```python
from build123d import *

# Parameters (mm, degrees)
SKETCH1_W             = 88.9
SKETCH1_H             = 38.1
BOSS_EXTRUDE1_DEPTH   = 12.7
SKETCH2_W             = 19.05
SKETCH2_H             = 25.4
CUT_EXTRUDE2_DEPTH    = 50.99995
SKETCH5_W             = 31.496
SKETCH5_H             = 31.75
CUT_EXTRUDE3_DEPTH    = 50.99995
BOSS_EXTRUDE2_START   = -6.35
BOSS_EXTRUDE2_DEPTH   = 6.35
SKETCH7_W             = 6.604
SKETCH7_H             = 6.604
CUT_EXTRUDE4_DEPTH    = 1.27
F_4_40_TAPPED_HOLE2_D = 2.2606
F_8_32_TAPPED_HOLE1_D = 3.4544
SKETCH20_R            = 1.5875
CUT_EXTRUDE5_DEPTH    = 1.27
FILLET3_R             = 3.175
SKETCH21_W            = 6.35
SKETCH21_H            = 12.7
CUT_EXTRUDE6_DEPTH    = 6.35
FILLET4_R             = 3.175
FILLET5_R             = 3.175
FILLET6_R             = 3.175
FILLET7_R             = 3.175


# Read off the part's stored shape, not the designer's step: Boss-Extrude2
with BuildPart() as part:
    # Sketch1 → Boss-Extrude1 (new body)
    with BuildSketch(Plane(origin=(0, 0, 0), x_dir=(1, 0, 0), z_dir=(0, 1, 0))):
        Rectangle(SKETCH1_W, SKETCH1_H)
    extrude(amount=-BOSS_EXTRUDE1_DEPTH)

    # Sketch2 → Cut-Extrude2 (cut, through all)
    with BuildSketch(Plane(origin=(0, 0, 0), x_dir=(1, 0, 0), z_dir=(0, 1, 0))):
        with Locations((-34.925, -6.35)):
            Rectangle(SKETCH2_W, SKETCH2_H)
        with Locations((34.925, -6.35)):
            Rectangle(SKETCH2_W, SKETCH2_H)
    extrude(amount=-CUT_EXTRUDE2_DEPTH, mode=Mode.SUBTRACT)

    # Sketch5 → Cut-Extrude3 (cut, through all)
    with BuildSketch(Plane(origin=(0, 0, 0), x_dir=(1, 0, 0), z_dir=(0, 1, 0))):
        with Locations((0, -3.175)):
            Rectangle(SKETCH5_W, SKETCH5_H)
    extrude(amount=-CUT_EXTRUDE3_DEPTH, mode=Mode.SUBTRACT)

    # Boss-Extrude2 outline → Boss-Extrude2 (cut)
    with BuildSketch(Plane.XZ.offset(12.7).offset(BOSS_EXTRUDE2_START)):
        Polygon((-25.4, 19.05), (-25.4, -19.05), (25.4, -19.05), (25.4, 19.05), (15.748, 19.05), (15.748, -12.7), (-15.748, -12.7), (-15.748, 19.05), align=None)
    extrude(amount=BOSS_EXTRUDE2_DEPTH, mode=Mode.SUBTRACT)

    # Sketch7 → Cut-Extrude4 (cut)
    with BuildSketch(Plane(origin=(0, 0, 0), x_dir=(1, 0, 0), z_dir=(0, 1, 0))):
        with Locations((-19.05, -15.748)):
            Rectangle(SKETCH7_W, SKETCH7_H)
        with Locations((19.05, -15.748)):
            Rectangle(SKETCH7_W, SKETCH7_H)
    extrude(amount=-CUT_EXTRUDE4_DEPTH, mode=Mode.SUBTRACT)

    # #4-40 Tapped Hole2 (through all)
    with Locations(Plane(origin=(-19.05, -1.27, 15.748), x_dir=(0, 0, 1), z_dir=(0, 1, 0))):
        with Locations((0, 0), (0, 38.1)):
            Hole(F_4_40_TAPPED_HOLE2_D / 2)

    # #8-32 Tapped Hole1 (through all)
    with Locations(Plane(origin=(-38.1, -6.35, -6.35), x_dir=(1, 0, 0), z_dir=(0, 0, 1))):
        with Locations((0, 0), (76.2, 0)):
            Hole(F_8_32_TAPPED_HOLE1_D / 2)

    # Sketch20 → Cut-Extrude5 (cut)
    with BuildSketch(Plane(origin=(0, 0, 0), x_dir=(1, 0, 0), z_dir=(0, 1, 0))):
        with Locations((-22.352, -12.446)):
            Circle(SKETCH20_R)
        with Locations((22.352, -12.446)):
            Circle(SKETCH20_R)
    extrude(amount=-CUT_EXTRUDE5_DEPTH, mode=Mode.SUBTRACT)

    # Fillet3
    fillet3_edges = [part.edges().sort_by_distance(p)[0] for p in [
        (15.748, -3.175, -12.7),
        (-15.748, -3.175, -12.7),
    ]]
    fillet(fillet3_edges, radius=FILLET3_R)

    # Sketch21 → Cut-Extrude6 (cut)
    with BuildSketch(Plane.XZ.offset(12.7)):
        with Locations((-28.575, -12.7)):
            Rectangle(SKETCH21_W, SKETCH21_H)
        with Locations((28.575, -12.7)):
            Rectangle(SKETCH21_W, SKETCH21_H)
    extrude(amount=-CUT_EXTRUDE6_DEPTH, mode=Mode.SUBTRACT)

    # Fillet4
    fillet4_edges = [part.edges().sort_by_distance(p)[0] for p in [
        (-31.75, -6.35, -12.7),
    ]]
    fillet(fillet4_edges, radius=FILLET4_R)

    # Fillet5
    fillet5_edges = [part.edges().sort_by_distance(p)[0] for p in [
        (31.75, -6.35, -12.7),
    ]]
    fillet(fillet5_edges, radius=FILLET5_R)

    # Fillet6
    fillet6_edges = [part.edges().sort_by_distance(p)[0] for p in [
        (-25.4, -3.175, -6.35),
    ]]
    fillet(fillet6_edges, radius=FILLET6_R)

    # Fillet7
    fillet7_edges = [part.edges().sort_by_distance(p)[0] for p in [
        (25.4, -3.175, -6.35),
    ]]
    fillet(fillet7_edges, radius=FILLET7_R)


solid = part.part
```
Geometry: final body of the model. Coordinates: model frame, mm. A direction names the side the tool comes from. Round coordinates to 2 decimals unless told otherwise and drop trailing zeros. Loops run counter-clockwise (first coordinate to the right, second up) from the corner with the lowest first, then second, coordinate; pieces in that order, holes last. Notation, with made-up numbers: (58.5, 89.5) -> (103.5, 89.5) arc R19 cw to (103.5, 119.5) -> close; hole circle Ø5 at (40, 15.25). An arc over 180 degrees is marked (long way). Use one line per item in the form item = value. Start each with the question number.
1) Section D-D on y = -11. Output: boundary loops of the cut face in (x, z), then the cut area to 3 significant figures.
2) Section A-A on y = -2.25. Output: boundary loops of the cut face in (x, z) (3 decimals), then the cut area to 3 significant figures.
3) Section B-B on x = -19.05. Output: boundary loops of the cut face in (y, z).
4) Draft query along Z for faces 1 (the cylindrical face through (19.814, -3.846, 16.581)), 2 (the flat face through (-1, -5, -19.05)), 3 (the cylindrical face through (-23.44, -0.63, 11.29)), 4 (the cylindrical face through (-26.35, -3.22, -5.44)). Return one class per face: released by +Z, released by -Z, zero draft, split by the parting line, or undercut.
5) Section C-C on z = -14.5. Output: boundary loops of the cut face in (x, y) (3 decimals).
6) Line query: L1, parallel to X at y = -3.75, z = 7; L2, parallel to X at y = -5, z = -10.5; L3, parallel to Y at x = 38.1, z = -11.5. Output: solid intervals per line, ascending.
7) First-contact query: P1, Ø1, axis at y = -1, z = 17.5, coming from the -X side; P2, Ø2.5, axis at x = -19, z = 13.5, coming from the +Y side; P3, Ø3, axis at x = 24.5, z = 5, coming from the -Y side; P4, Ø5, axis at y = -3, z = 3.5, coming from the +X side. Flat tips, straight axial feed; report the tip coordinate or a pass-through.
8) Access query for faces 5 (the cylindrical face through (-30.8, -7.26, -12.61)), 6 (the cylindrical face through (23.51, -0.63, 11.36)), 7 (the flat face through (-36.6, -4.8, -6.35)), 8 (the flat face through (25.4, -3, 8)), 9 (the flat face through (15.748, -3, 5)). Directions: +Z, -Z, +X, -X, +Y, -Y. A direction counts if a zero-diameter tool reaches every point of the face in a straight line with its end or side. Return the directions, or none.
Response:
q1.outline = (-44.45, -19.05) -> (-31.75, -19.05) -> (-31.75, -6.35) -> (-44.45, -6.35) -> close; (31.75, -19.05) -> (44.45, -19.05) -> (44.45, -6.35) -> (31.75, -6.35) -> close
q1.area = 323 mm^2
q2.outline = (-44.45, -19.05) -> (44.45, -19.05) -> (44.45, -6.35) -> (28.575, -6.35) arc R3.175 cw to (25.4, -3.175) -> (25.4, 19.05) -> (15.748, 19.05) -> (15.748, -9.525) arc R3.175 cw to (12.573, -12.7) -> (-12.573, -12.7) arc R3.175 cw to (-15.748, -9.525) -> (-15.748, 19.05) -> (-25.4, 19.05) -> (-25.4, -3.175) arc R3.175 cw to (-28.575, -6.35) -> (-44.45, -6.35) -> close; hole circle Ø2.261 at (-19.05, 15.748); hole circle Ø2.261 at (19.05, 15.748)
q2.area = 1,420 mm^2
q3.outline = (-6.35, -19.05) -> (0, -19.05) -> (0, 12.45) -> (-1.27, 12.45) -> (-1.27, 14.62) -> (-6.35, 14.62) -> close; (-6.35, 16.88) -> (-1.27, 16.88) -> (-1.27, 19.05) -> (-6.35, 19.05) -> close
q4.face_1 = undercut
q4.face_2 = released by -Z
q4.face_3 = undercut
q4.face_4 = released by +Z
q5.outline = (-44.45, -12.7) -> (-31.75, -12.7) -> (-31.75, -9.525) arc R3.175 cw to (-28.575, -6.35) -> (28.575, -6.35) arc R3.175 cw to (31.75, -9.525) -> (31.75, -12.7) -> (44.45, -12.7) -> (44.45, 0) -> (-44.45, 0) -> close; hole circle Ø3.454 at (-38.1, -6.35); hole circle Ø3.454 at (38.1, -6.35)
q6.L1 = -25.4 to -15.75, 15.75 to 25.4
q6.L2 = -44.45 to -39.18, -37.02 to -15.59, 15.59 to 37.02, 39.18 to 44.45
q6.L3 = -12.7 to -8.08, -4.62 to 0
q7.P1 = -25.4
q7.P2 = 0
q7.P3 = -6.35
q7.P4 = 25.4
q8.face_5 = +Z, -Z, -Y
q8.face_6 = +Y
q8.face_7 = +Z, -X, +Y, -Y
q8.face_8 = +Z, +X, +Y, -Y
q8.face_9 = +Z, +Y, -Y
